Can you work these out from the model? Positions are in its coordinate system, mm. A direction names the side the tool comes from. Round coordinates to 2 decimals unless told otherwise and drop trailing zeros. Loops run counter-clockwise (first coordinate to the right, second up) from the corner with the lowest first, then second, coordinate; pieces in that order, holes last.
from build123d import *

# Parameters (mm, degrees)
F0_R     = 25.4
F1_DEPTH = 38.1
F2_R     = 19.05
F3_DEPTH = 76.201
F4_SIZE  = 2.54
F5_T     = -0.254


with BuildPart() as f1:
    # F0 (on Front) → F1 (new body, symmetric)
    with BuildSketch(Plane.XZ):
        Circle(F0_R)
    extrude(amount=F1_DEPTH, both=True)

    # F2 (on face) → F3 (cut, through all)
    with BuildSketch(Plane.XZ.offset(38.1)):
        Circle(F2_R)
    extrude(amount=-F3_DEPTH, mode=Mode.SUBTRACT)

    # F4
    f4_edges = [f1.edges().sort_by_distance(p)[0] for p in [
        (-25.4, -38.1, 0),
    ]]
    chamfer(f4_edges, length=F4_SIZE)

    # F5
    f5_openings = [f1.faces().sort_by_distance(p)[0] for p in [
        (-24.68158, 38.1, 0),
    ]]
    offset(amount=F5_T, openings=f5_openings)


solid = f1.part
(1) Will these pins go through, and if not, where does the flat tip stop? P1, Ø6, axis at y = 27, z = 5, coming from the -X side; P2, Ø5, axis at x = -9, y = -11, coming from the -Z side; P3, Ø3, axis at y = 11, z = -6, coming from the -X side; P4, Ø8, axis at y = -22, z = -3.5, coming from the +X side.
Worked answers:
P1: stops at x = -25.32
P2: stops at z = -24.55
P3: stops at x = -25
P4: stops at x = 25.4
(2) For faces 5 (the conical face through (-4.982, -37.977, -22.437)), 6 (the flat face through (-10, -37.846, -17)), which set-ups out of +Z, -Z, +X, -X, +Y, -Y let a thin tool reach every point of the face, with its end or its side?
Worked answers:
face 5: -Y
face 6: +Y
(3) If we mould it in two halves opening along X, with no side actions, what happens to faces 1 (the cylindrical face through (-4.185, -0.405, -18.845)), 2 (the cylindrical face through (-5.45, 0.81, -24.55)), 3 (the flat face through (-9, -38.1, 17)), 4 (the cylindrical face through (-5.506, 0.754, -24.796))? For each: released by +X, released by -X, zero draft, split by the parting line, or undercut.
Worked answers:
face 1: undercut
face 2: undercut
face 3: zero draft
face 4: split by the parting line
(4) If we section it at B-B, the plane x = 0: List the corners of the cut face in (y, z) for me, then the cut area to 3 significant figures.
Worked answers:
outline: (-38.1, -22.86) - (-35.56, -25.4) - (38.1, -25.4) - (38.1, -25.15) - (-35.45, -25.15) - (-37.85, -22.75) - (-37.85, -19.3) - (38.1, -19.3) - (38.1, -19.05) - (-38.1, -19.05) - close; (-38.1, 19.05) - (38.1, 19.05) - (38.1, 19.3) - (-37.85, 19.3) - (-37.85, 22.75) - (-35.45, 25.15) - (38.1, 25.15) - (38.1, 25.4) - (-35.56, 25.4) - (-38.1, 22.86) - close
area: 79.7 mm2
(5) If we section it at C-C, the plane y = -4: List the corners of the cut face in (x, z) for me, then the cut area to 3 significant figures.
Worked answers:
outline: circle Ø50.8 at (0, 0); circle Ø38.61 at (0, 0); hole circle Ø50.29 at (0, 0); hole circle Ø38.1 at (0, 0)
area: 70.9 mm2
(6) If I drill on line 1 (Z direction, x = 0, y = 3); line 2 (Z direction, x = 12, y = 23); line 3 (X direction, y = 31, z = -8), over which ranges is the centre line in solid material (lowest first)?
Worked answers:
line 1: z = -25.4 to -25.15, -19.3 to -19.05, 19.05 to 19.3, 25.15 to 25.4
line 2: z = -22.39 to -22.1, -15.12 to -14.8, 14.8 to 15.12, 22.1 to 22.39
line 3: x = -24.11 to -23.84, -17.57 to -17.29, 17.29 to 17.57, 23.84 to 24.11
(7) If we section it at A-A, the plane z = 0: List the corners of the cut face in (x, y) for me, then the cut area to 3 significant figures.
Worked answers:
outline: (-25.4, -35.56) - (-22.86, -38.1) - (-19.05, -38.1) - (-19.05, 38.1) - (-19.3, 38.1) - (-19.3, -37.85) - (-22.75, -37.85) - (-25.15, -35.45) - (-25.15, 38.1) - (-25.4, 38.1) - close; (19.05, -38.1) - (22.86, -38.1) - (25.4, -35.56) - (25.4, 38.1) - (25.15, 38.1) - (25.15, -35.45) - (22.75, -37.85) - (19.3, -37.85) - (19.3, 38.1) - (19.05, 38.1) - close
area: 79.7 mm2
